Geometry: final body of the model. Coordinates: model frame, mm. A direction names the side the tool comes from. Round coordinates to 2 decimals unless told otherwise and drop trailing zeros. Loops run counter-clockwise (first coordinate to the right, second up) from the corner with the lowest first, then second, coordinate; pieces in that order, holes last. Notation, with made-up numbers: (-23.75, 61.25) - (24.25, 61.25) arc R22 ccw to (24.25, 76.25) - close; hole circle Ø9 at (82.5, -10). An arc over 180 degrees is marked (long way). Answer as a JSON object with one key per item and string values. Group by question number.
Item 1: Reachability of faces 5 (the face through (29, -0.475, 5)), 6 (the face through (0.2, 47.5, 20.5)), 7 (the face through (29.34, 47.52, 45.45)) from +Z, -Z, +X, -X, +Y, -Y: full face, straight path, thin tool, end or side. Return the list, or none.
Item 2: Section C-C (z = 35). Return the cut outline in (x, y) (3 decimals).
Item 3: Section D-D (x = -7.25). Return the cut outline in (y, z) (3 decimals), plus the area to 3 significant figures.
Item 4: Section A-A (x = 0). Return the cut outline in (y, z) (3 decimals).
Item 5: Section B-B (y = 42). Return the cut outline in (x, z).
Item 6: First-contact query: pin 1 (12 mm diameter, centred on y = 13, z = 32, fed in from +X); pin 2 (14 mm diameter, centred on x = 23.8, z = 47.75, fed in from -Y) (3 decimals); pin 3 (1 mm diameter, centred on x = -3.5, z = 42.5, fed in from +Y) (3 decimals). Flat tips, straight axial feed; report the tip coordinate or a pass-through.
Item 7: Draft query along Z for faces 1 (the face through (31.25, 42, 16)), 2 (the face through (-29.215, 47.517, 45.165)), 3 (the face through (0.527, 42.503, 39.016)), 4 (the face through (25.372, 47.517, 56.857)). Return one class per face: released by +Z, released by -Z, zero draft, split by the parting line, or undercut.
Item 8: Line query: line 1 (Y direction, x = -7.25, z = 5.5) (3 decimals); line 2 (Y direction, x = 5, z = 2) (3 decimals); line 3 (Z direction, x = 0, y = 41.75). Output: solid intervals per line, ascending.
```python
from build123d import *

# Parameters (mm, degrees)
F0_R            = 1.7
F1_DEPTH        = 10
F3_DEPTH        = 50
F4_R            = 4.05
F5_DEPTH        = 6
F6_R            = 4.05
F7_DEPTH        = 25
F8_DEPTH        = 5
F9_DEPTH        = 5
F11_DEPTH       = 5
F13_D           = 3.2
F13_CBORE_D     = 12
F13_CBORE_DEPTH = 6


with BuildPart() as f1:
    # F0 (on Top) → F1 (new body)
    with BuildSketch(Plane.XY):
        with BuildLine():
            Line((26.25, 50.475), (-26.25, 50.475))
            Line((-26.25, 50.475), (-26.25, -50.475))
            Line((-26.25, -50.475), (10.25, -50.475))
            ThreePointArc((10.25, -50.475), (13.7855339059, -49.0105339059), (15.25, -45.475))
            Line((15.25, -45.475), (15.25, -10.475))
            ThreePointArc((15.25, -10.475), (16.7144660941, -6.9394660941), (20.25, -5.475))
            Line((20.25, -5.475), (21.25, -5.475))
            ThreePointArc((21.25, -5.475), (24.7855339059, -4.0105339059), (26.25, -0.475))
            Line((26.25, -0.475), (26.25, 50.475))
        make_face()
        with Locations((-7.25, -40.338)):
            Circle(F0_R, mode=Mode.SUBTRACT)
        with Locations((-7.25, -13.738)):
            Circle(F0_R, mode=Mode.SUBTRACT)
        with Locations((5.25, -40.338)):
            Circle(F0_R, mode=Mode.SUBTRACT)
        with Locations((5.25, -13.738)):
            Circle(F0_R, mode=Mode.SUBTRACT)
    extrude(amount=F1_DEPTH)

    # F2 (on face) → F3 (join)
    with BuildSketch(Plane.XY.offset(10)):
        Polygon((26.25, 50.475), (-26.25, 50.475), (-26.25, 40.475), (-21.25, 40.475), (26.25, 40.475), align=None)
    extrude(amount=F3_DEPTH)

    # F4 (on face) → F5 (cut)
    with BuildSketch(Plane(origin=(0, 50.475, 0), x_dir=(-1, 0, 0), z_dir=(0, 1, 0))):
        with BuildLine():
            Line((13.1008645921, 28.7857142857), (23.2653284998, 50.2142857143))
            ThreePointArc((23.2653284998, 50.2142857143), (24.9764267273, 54.9857675702), (25.7196422992, 60))
            Line((25.7196422992, 60), (-25.7196422992, 60))
            ThreePointArc((-25.7196422992, 60), (-24.9764267273, 54.9857675702), (-23.2653284998, 50.2142857143))
            Line((-23.2653284998, 50.2142857143), (-13.1008645921, 28.7857142857))
            ThreePointArc((-13.1008645921, 28.7857142857), (0, 20.5), (13.1008645921, 28.7857142857))
        make_face()
        with Locations((0, 35)):
            Circle(F4_R, mode=Mode.SUBTRACT)
        with Locations((0, 35)):
            Circle(F4_R)
    extrude(amount=-F5_DEPTH, mode=Mode.SUBTRACT)

    # F6 (on face) → F7 (cut)
    with BuildSketch(Plane(origin=(0, 50.475, 0), x_dir=(-1, 0, 0), z_dir=(0, 1, 0))):
        with Locations((0, 35)):
            Circle(F6_R)
        with BuildLine():
            Line((-22.5965488101, 48.8043743327), (-22.2220881702, 48.0149419886))
            ThreePointArc((-22.2220881702, 48.0149419886), (-22.3543873554, 48.4357142857), (-22.5965488101, 48.8043743327))
        make_face()
        with BuildLine():
            ThreePointArc((-22.5965488101, 48.8043743327), (-25.29758504, 47.1867602215), (-22.2, 47.75))
            ThreePointArc((-22.2, 47.75), (-22.2055316046, 47.8829305689), (-22.2220881702, 48.0149419886))
            Line((-22.2220881702, 48.0149419886), (-22.5965488101, 48.8043743327))
        make_face()
        with BuildLine():
            ThreePointArc((22.5965488101, 48.8043743327), (22.3543873554, 48.4357142857), (22.2220881702, 48.0149419886))
            Line((22.2220881702, 48.0149419886), (22.5965488101, 48.8043743327))
        make_face()
        with BuildLine():
            Line((22.5965488101, 48.8043743327), (22.2220881702, 48.0149419886))
            ThreePointArc((22.2220881702, 48.0149419886), (23.6670694311, 46.1555316046), (25.4, 47.75))
            ThreePointArc((25.4, 47.75), (24.3632397785, 49.24758504), (22.5965488101, 48.8043743327))
        make_face()
    extrude(amount=-F7_DEPTH, mode=Mode.SUBTRACT)

    # F8 (add): a face of the model
    f8_faces = [f1.faces().sort_by_distance(p)[0] for p in [
        (-26.25, 49.3006532667, 30),
    ]]
    extrude(f8_faces, amount=F8_DEPTH)

    # F9 (add): a face of the model
    f9_faces = [f1.faces().sort_by_distance(p)[0] for p in [
        (26.25, 0.3121405529, 5),
    ]]
    extrude(f9_faces, amount=F9_DEPTH)

    # F10 (on face) → F11 (join)
    with BuildSketch(Plane(origin=(-31.25, 0, 0), x_dir=(0, -1, 0), z_dir=(-1, 0, 0))):
        Polygon((50.475, 10), (-40.475, 60), (-40.475, 10), align=None)
    extrude(amount=-F11_DEPTH)

    # F13 (through all)
    with Locations(Plane(origin=(0, 50.475, 0), x_dir=(-1, 0, 0), z_dir=(0, 1, 0))):
        with Locations((-23.8, 47.75), (23.8, 47.75)):
            CounterBoreHole(F13_D / 2, F13_CBORE_D / 2, F13_CBORE_DEPTH)


solid = f1.part
```
Values:
{
 "1": {"face 5": "+Z, -Z, +X, -Y", "face 6": "+Z, +Y", "face 7": "+Y"},
 "2": {"outline": "(-31.25, -5) - (-26.25, -5) - (-26.25, 40.475) - (-4.05, 40.475) - (-4.05, 44.475) - (-16.049, 44.475) - (-16.049, 50.475) - (-31.25, 50.475) - close; (4.05, 40.475) - (31.25, 40.475) - (31.25, 50.475) - (16.049, 50.475) - (16.049, 44.475) - (4.05, 44.475) - close"},
 "3": {"outline": "(-50.475, 0) - (-42.038, 0) - (-42.038, 10) - (-50.475, 10) - close; (-38.638, 0) - (-15.438, 0) - (-15.438, 10) - (-38.638, 10) - close; (-12.038, 0) - (50.475, 0) - (50.475, 22.443) - (44.475, 22.443) - (44.475, 60) - (40.475, 60) - (40.475, 10) - (-12.038, 10) - close", "area": "1,220 mm^2"},
 "4": {"outline": "(-50.475, 0) - (50.475, 0) - (50.475, 20.5) - (44.475, 20.5) - (44.475, 30.95) - (40.475, 30.95) - (40.475, 10) - (-50.475, 10) - close; (40.475, 39.05) - (44.475, 39.05) - (44.475, 60) - (40.475, 60) - close"},
 "5": {"outline": "(-31.25, 0) - (31.25, 0) - (31.25, 60) - (-31.25, 60) - close; hole circle Ø3.2 at (-23.8, 47.75); hole circle Ø8.1 at (0, 35); hole circle Ø3.2 at (23.8, 47.75)"},
 "6": {"pin 1": "stops at x = -26.25", "pin 2": "stops at y = 40.475", "pin 3": "stops at y = 44.475"},
 "7": {"face 1": "zero draft", "face 2": "undercut", "face 3": "undercut", "face 4": "released by +Z"},
 "8": {"line 1": "y = -50.475 to -42.038, -38.638 to -15.438, -12.038 to 50.475", "line 2": "y = -50.475 to -42.02, -38.656 to -15.42, -12.056 to 50.475", "line 3": "z = 0 to 30.95, 39.05 to 60"}
}
